Check sheet for the modelled part. Datum: model origin and axes. Units: mm. A direction names the side the tool comes from. Round coordinates to 2 decimals unless told otherwise and drop trailing zeros. Write each loop counter-clockwise with the first axis right and the second up, starting at its lowest first coordinate (ties: lowest second). Pieces come first, ordered by that corner, then holes. Notation, with made-up numbers: (82, 19.25) - (95, 19.25) arc R28 ccw to (95, 43.25) - close; hole circle Ø10 at (18, 29). An arc over 180 degrees is marked (long way). Answer as a JSON object with one key per item and string values. Group by question number.
Item 1: Sectioned sample at B-B on y = 38. Record the boundary of the cut face in (x, z), plus the area to 3 significant figures.
Item 2: Gauge pin test, flat ends, axial feed: P1, Ø5.5, axis at x = 10, y = 41.5, coming from the +Z side; P2, Ø0.5, axis at x = 13.5, z = 8.5, coming from the +Y side; P3, Ø10, axis at x = 8, y = 24, coming from the -Z side; P4, Ø0.8, axis at x = 14.5, z = 8.5, coming from the +Y side. Record the tip position at first contact, or that the pin passes through.
Item 3: Release check for a two-part mould opening along X. For faces 1 (the flat face through (13, 43, 6)), 2 (the flat face through (12.7, 14.522, 8.5)) record: pulls with the +X half, pulls with the -X half, needs draft (parallel to the pull), parting line crosses it, or undercut.
Item 4: Set-up check for faces 3 (the flat face through (13, 0, 4)), 4 (the flat face through (12.4, 6.622, 8.5)): record each of +Z, -Z, +X, -X, +Y, -Y from which the full face is reachable in a straight line by a thin tool's end or side.
Item 5: Thickness scan on line 1 (Y direction, x = 1.75, z = 7.75); line 2 (Y direction, x = 8, z = 7.5). Record the ranges inside material, lowest first.
Item 6: Sectioned sample at C-C on z = 7.25. Record the boundary of the cut face in (x, y).
Item 7: Sectioned sample at A-A on x = 1.5. Record the boundary of the cut face in (y, z).
Autodesk Inventor part; units mm, degrees
ref_plane "YZ Plane" through (0, 0, 0) normal (1, 0, 0) x (0, 1, 0)
ref_plane "XZ Plane" through (0, 0, 0) normal (0, 1, 0) x (-1, 0, 0)
ref_plane "XY Plane" through (0, 0, 0) normal (0, 0, 1) x (1, 0, 0)
sketch "Sketch1" plane through (0, 0, 0) normal (0, 0, 1) x (1, 0, 0)
  line L0 (0, 0) -> (26, 0)
  line L1 (26, 0) -> (26, 45)
  line L2 (26, 45) -> (0, 45)
  line L3 (0, 45) -> (0, 0)
  dimension "d0" = 26
  dimension "d1" = 45
extrude "Extrusion1" add sketch "Sketch1" along normal blind 6
sketch "Sketch2" plane through (0, 0, 6) normal (0, 0, 1) x (1, 0, 0)
  line L0 (26, 0) -> (26, 45)
  line L1 (0, 0) -> (26, 0)
  line L2 (26, 0) -> (26, 35)
  line L3 (26, 35) -> (0, 35)
  line L4 (0, 35) -> (0, 0)
  dimension "d4" = 35
extrude "Extrusion2" add sketch "Sketch2" along normal blind 3
draft "FaceDraft1" angle 60 pull direction (0, 0, 1) faces at (17.3333, 35, 7) fixed edges at (13, 35, 9)
sketch "Sketch3" plane through (0, 0, 9) normal (0, 0, 1) x (1, 0, 0)
  line L0 (10.2597, 5.4477) -> (10.2597, 19.6754) construction
  line L1 (10.2597, 19.6754) -> (17.2769, 19.6754) construction
  line L2 (17.2769, 19.6754) -> (17.2769, 5.4477) construction
  line L3 (17.2769, 5.4477) -> (10.2597, 5.4477) construction
  line L4 (0, 0) -> (26, 0)
  line L5 (13, 0) -> (13, 5.1104)
  line L6 (15.2597, 5.9584) -> (10.2597, 5.9584)
  line L7 (10.2597, 5.9584) -> (10.2597, 6.6215)
  line L8 (10.2597, 6.6215) -> (14.669, 6.6215)
  line L9 (14.669, 6.6215) -> (14.669, 9.0834)
  line L10 (14.669, 9.0834) -> (15.2597, 9.0834)
  line L11 (15.2597, 9.0834) -> (15.2597, 5.9584)
  line L12 (15.2597, 9.7961) -> (11.6354, 9.7961)
  line L13 (11.6354, 9.7961) -> (11.6354, 10.4096)
  line L14 (11.6354, 10.4096) -> (15.2597, 10.4096)
  line L15 (15.2597, 10.4096) -> (15.2597, 9.7961)
  line L16 (10.9647, 9.7961) -> (10.2597, 9.7961)
  line L17 (10.2597, 9.7961) -> (10.2597, 10.4096)
  line L18 (10.2597, 10.4096) -> (10.9647, 10.4096)
  line L19 (10.9647, 10.4096) -> (10.9647, 9.7961)
  line L20 (13.7581, 11.0994) -> (13.1408, 11.0994)
  line L21 (13.1408, 11.0994) -> (13.1408, 12.9897)
  line L22 (13.1408, 12.9897) -> (13.7581, 12.9897)
  line L23 (13.7581, 12.9897) -> (13.7581, 11.0994)
  line L24 (15.2597, 13.8586) -> (10.2597, 13.8586)
  line L25 (10.2597, 13.8586) -> (10.2597, 14.5217)
  line L26 (10.2597, 14.5217) -> (15.2597, 14.5217)
  line L27 (15.2597, 14.5217) -> (15.2597, 13.8586)
  spline S0 degree 2 poles (13.4456, 15.3791) (12.4433, 15.3791) (11.9593, 15.9394) knots 0 0 0 1 1 1
  spline S1 degree 2 poles (11.9593, 15.9394) (11.5554, 16.4043) (11.5554, 17.075) knots 0 0 0 1 1 1
  spline S2 degree 2 poles (11.5554, 17.075) (11.5554, 17.822) (12.5348, 18.7709) (13.3961, 18.7709) knots 0 0 0 1 2 2 2
  spline S3 degree 2 poles (13.3961, 18.7709) (14.0935, 18.7709) (14.8976, 18.3517) (15.3397, 17.5514) (15.3397, 17.075) knots 0 0 0 1 2 3 3 3
  spline S4 degree 2 poles (15.3397, 17.075) (15.3397, 16.3166) (14.3641, 15.3791) (13.4456, 15.3791) knots 0 0 0 1 2 2 2
  spline S5 degree 2 poles (13.4494, 16.0118) (14.143, 16.0118) (14.8366, 16.6177) (14.8366, 17.075) knots 0 0 0 1 2 2 2
  spline S6 degree 2 poles (14.8366, 17.075) (14.8366, 17.5323) (14.1392, 18.1383) (13.4266, 18.1383) knots 0 0 0 1 2 2 2
  spline S7 degree 2 poles (13.4266, 18.1383) (12.7558, 18.1383) (12.0622, 17.5285) (12.0622, 17.075) knots 0 0 0 1 2 2 2
  spline S8 degree 2 poles (12.0622, 17.075) (12.0622, 16.6177) (12.752, 16.0118) (13.4494, 16.0118) knots 0 0 0 1 2 2 2
  line L28 (15.2597, 19.4912) -> (11.6354, 19.4912)
  line L29 (11.6354, 19.4912) -> (11.6354, 20.0438)
  line L30 (11.6354, 20.0438) -> (12.1499, 20.0438)
  spline S9 degree 2 poles (12.1499, 20.0438) (11.5554, 20.4439) (11.5554, 21.1947) knots 0 0 0 1 1 1
  spline S10 degree 2 poles (11.5554, 21.1947) (11.5554, 21.5224) (11.7917, 22.0712) (12.1728, 22.3456) (12.4357, 22.399) knots 0 0 0 1 2 3 3 3
  spline S11 degree 2 poles (12.4357, 22.399) (12.6072, 22.4333) (13.034, 22.4333) knots 0 0 0 1 1 1
  line L31 (13.034, 22.4333) -> (15.2597, 22.4333)
  line L32 (15.2597, 22.4333) -> (15.2597, 21.8197)
  line L33 (15.2597, 21.8197) -> (13.0569, 21.8197)
  spline S12 degree 2 poles (13.0569, 21.8197) (12.6834, 21.8197) (12.31, 21.6749) (12.0889, 21.3128) (12.0889, 21.0651) knots 0 0 0 1 2 3 3 3
  spline S13 degree 2 poles (12.0889, 21.0651) (12.0889, 20.6726) (12.5882, 20.1048) (13.2818, 20.1048) knots 0 0 0 1 2 2 2
  line L34 (13.2818, 20.1048) -> (15.2597, 20.1048)
  line L35 (15.2597, 20.1048) -> (15.2597, 19.4912)
extrude "Extrusion3" cut sketch "Sketch3" against normal blind 1
properties part number "Li-IonBattery"
Completed:
{
 "1": {"outline": "(0, 0) - (26, 0) - (26, 7.27) - (0, 7.27) - close", "area": "189 mm²"},
 "2": {"P1": "z = 6.83", "P2": "y = 36.3", "P3": "z = 0", "P4": "y = 36.56"},
 "3": {"face 1": "needs draft", "face 2": "undercut"},
 "4": {"face 3": "+Z, -Z, +X, -X, -Y", "face 4": "+Z"},
 "5": {"line 1": "0 to 37.17", "line 2": "0 to 37.6"},
 "6": {"outline": "(0, 0) - (26, 0) - (26, 38.03) - (0, 38.03) - close"},
 "7": {"outline": "(0, 0) - (45, 0) - (45, 6) - (40.2, 6) - (35, 9) - (0, 9) - close"}
}
